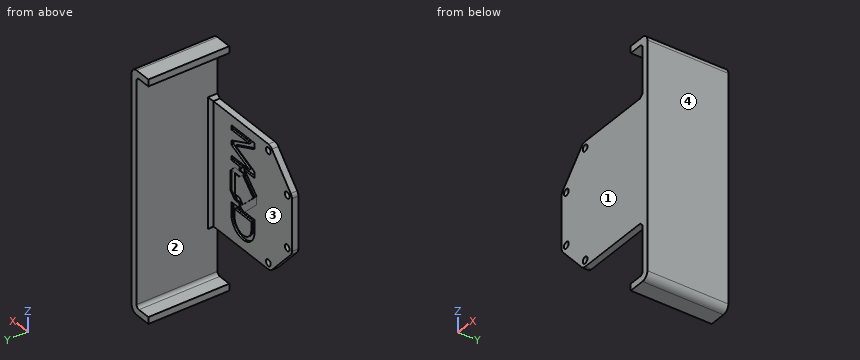
Autodesk Inventor part; units mm, degrees
ref_plane "YZ Plane" through (0, 0, 0) normal (1, 0, 0) x (0, 1, 0)
ref_plane "XZ Plane" through (0, 0, 0) normal (0, 1, 0) x (-1, 0, 0)
ref_plane "XY Plane" through (0, 0, 0) normal (0, 0, 1) x (1, 0, 0)
sketch "Sketch1" plane through (0, 0, 0) normal (0, 1, 0) x (-1, 0, 0)
  line L0 (0, 34) -> (16, 16) construction
  line L1 (18.9896, 18.6575) -> (2.9896, 36.6575)
  arc A0 (2.9896, 36.6575) -> (0, 38) centre (0, 34) ccw
  arc A1 (20, 16) -> (18.9896, 18.6575) centre (16, 16) ccw
  line L2 (16, 16) -> (16, -16) construction
  line L3 (20, -16) -> (20, 16)
  line L4 (16, -16) -> (0, -34) construction
  line L5 (2.9896, -36.6575) -> (18.9896, -18.6575)
  line L6 (0, 34) -> (-44.6053, 34) construction
  line L7 (0, 38) -> (-53, 38)
  line L8 (0, -34) -> (-49, -34) construction
  line L9 (-53, -38) -> (0, -38)
  line L10 (-49, 30.0008) -> (-49, -29.9992) construction
  line L11 (-53, 38) -> (-53, -38)
  arc A2 (18.9896, -18.6575) -> (20, -16) centre (16, -16) ccw
  arc A3 (0, -38) -> (2.9896, -36.6575) centre (0, -34) ccw
  point P0 (0, 0)
  point P1 (8, 25)
  point P2 (16, 0)
  point P3 (8, -25)
  point P4 (-24.1053, 34)
  point P5 (-24.5, -34)
  point P6 (-49, 0.0008)
  dimension "d1" = 34
  dimension "d2" = 32
  dimension "d3" = 16
  dimension "d4" = 16
  dimension "d6" = 8
  dimension "d12" = 4
  dimension "d13" = 4
  dimension "d15" = 4
  dimension "d17" = 68
  dimension "d18" = 76
  dimension "d19" = 73
  dimension "d21" = 20
  dimension "d40" = 76
  dimension "d41" = 53
extrude "Extrusion1" add sketch "Sketch1" along normal blind 4
sketch "Sketch2" plane through (0, 4, 0) normal (0, 1, 0) x (1, 0, 0)
  line L0 (-20, 16) -> (-20, -16)
  point P0 (0, 0)
  point P1 (0, -34)
  point P2 (-16, 16)
  point P3 (-16, -16)
  point P4 (0, 34)
  dimension "d31" = 34
  dimension "d33" = 20
  dimension "d34" = 16
  dimension "d35" = 4
  dimension "d36" = 16
  dimension "d37" = 4
  dimension "d38" = 20
  dimension "d39" = 34
hole "Hole1" at (0, 4, 34) at (-16, 4, -16) at (-16, 4, 16) at (0, 4, -34) direction (0, -1, 0) diameter 4 end through all
sketch "Sketch3" plane through (0, 4, 0) normal (0, 1, 0) x (1, 0, 0)
  line L0 (53, -70) -> (53, 70)
  line L1 (48.8, 70) -> (48.8, -70)
  line L2 (53, -38) -> (53, 38)
  arc A0 (53, 70) -> (48.8, 74.2) centre (48.8, 70) ccw
  arc A1 (48.8, -74.2) -> (53, -70) centre (48.8, -70) ccw
  line L3 (48.8, 74.2) -> (38.8, 74.2)
  line L4 (38.8, 74.2) -> (38.8, 70)
  line L5 (38.8, 70) -> (48.8, 70)
  line L6 (48.8, -74.2) -> (38.8, -74.2)
  line L7 (38.8, -74.2) -> (38.8, -70)
  line L8 (38.8, -70) -> (48.8, -70)
  point P0 (0, 0)
  dimension "d42" = 140
  dimension "d43" = 4.2
  dimension "d52" = 70
  dimension "d53" = 10
  dimension "d54" = 10
extrude "Extrusion2" add sketch "Sketch3" along normal blind 46 and the other way blind 4
chamfer "Chamfer1" distance 2 angle 45 3 edges at (48.8, 4, 0) (48.8, 2, 38) (48.8, 2, -38)
fillet "Fillet1" radius 2 1 edges at (48.8, 25, 70)
fillet "Fillet2" radius 2 1 edges at (48.8, 25, -70)
sketch "Sketch9" plane through (0, 4, 0) normal (0, 1, 0) x (1, 0, 0)
  line L0 (21.0218, -11.6451) -> (10.117, -0.7403)
  line L1 (10.117, -0.7403) -> (10.117, 4.4923)
  line L2 (10.117, 4.4923) -> (21.0218, 15.3971)
  line L3 (21.0218, 15.3971) -> (24.6218, 13.7645)
  line L4 (24.6218, 13.7645) -> (24.6218, 11.726)
  line L5 (24.6218, 11.726) -> (28.517, 11.726)
  line L6 (28.517, 11.726) -> (32.117, 8.126)
  line L7 (32.117, 8.126) -> (32.117, -4.374)
  line L8 (32.117, -4.374) -> (28.517, -7.974)
  line L9 (28.517, -7.974) -> (24.6218, -7.974)
  line L10 (24.6218, -7.974) -> (24.6218, -10.0125)
  line L11 (24.6218, -10.0125) -> (21.0218, -11.6451)
  line L12 (28.517, -4.374) -> (24.6218, -4.374)
  line L13 (24.6218, -4.374) -> (21.8025, -7.1932)
  line L14 (21.8025, -7.1932) -> (12.7333, 1.876)
  line L15 (12.7333, 1.876) -> (21.8025, 10.9453)
  line L16 (21.8025, 10.9453) -> (24.6218, 8.126)
  line L17 (24.6218, 8.126) -> (28.517, 8.126)
  line L18 (28.517, 8.126) -> (28.517, -4.374)
  line L19 (10.117, -0.7403) -> (24.6218, 13.7645)
  line L20 (24.6218, -10.0125) -> (10.117, 4.4923)
  line L21 (21.8025, -7.1932) -> (21.8025, 10.9453)
  line L22 (21.0218, -11.6451) -> (21.0218, 15.3971)
  line L23 (24.6218, -7.974) -> (21.0218, -7.974)
  line L24 (21.8025, -7.1932) -> (21.0218, -7.974)
  line L25 (32.117, -4.374) -> (28.517, -4.374)
  line L26 (32.117, 8.126) -> (28.517, 8.126)
  line L27 (24.6218, 11.726) -> (24.6218, 8.126)
  line L28 (28.517, 8.126) -> (28.517, 11.726)
  line L29 (21.0218, -7.974) -> (24.6218, -7.974)
  line L30 (21.8025, -7.1932) -> (21.0218, -7.974)
  line L31 (21.0218, -11.6451) -> (21.0218, -7.974)
  line L32 (12.7333, 1.876) -> (10.117, -0.7403)
  line L33 (21.8025, 10.9453) -> (24.6218, 13.7645)
  line L34 (28.517, -4.374) -> (32.117, -4.374)
  line L35 (0, -38) -> (46.8, -38)
  point P0 (-70, 0)
  point P1 (21.0218, -6.4125)
  dimension "d467" = 3.7
  dimension "d468" = 3.7
  dimension "d469" = 12.5
  dimension "d470" = 3.6
  dimension "d471" = 3.6
  dimension "d472" = 2.0385
  dimension "d473" = 3.6
  dimension "d474" = 22
  dimension "d475" = 3.6
  dimension "d523" = 30.026
extrude "Extrusion16" cut sketch "Sketch9" against normal blind 0.6 contours L22 L23 L20 L11 | L20 L23 L10 | L19 L4 L27 L16 | L25 L18 L26 L7 | L26 L28 L6
extrude "Extrusion19" cut sketch "Sketch9" against normal blind 0.3 contours L1 L20 L19 | L24 L20 L23 | L2 L22 L15 L20 | L23 L20 L13 L12 L25 L8 L9 | L3 L19 L15 L22
sketch "Sketch10" plane through (0, 4, 0) normal (0, 1, 0) x (1, 0, 0)
  line L0 (31.4873, 14.588) -> (11.8138, 14.588)
  line L1 (31.4873, 14.588) -> (31.4873, 22.6975)
  line L2 (11.8138, 22.8893) -> (11.8138, 14.588)
  line L3 (28.7873, 17.288) -> (28.7996, 22.3152)
  line L4 (28.7873, 17.288) -> (14.4873, 17.288)
  line L5 (14.4873, 17.288) -> (14.4873, 22.181)
  arc A0 (31.4873, 22.6975) -> (11.8138, 22.8893) centre (21.6443, 22.1561) ccw
  arc A1 (28.7996, 22.3152) -> (14.4873, 22.181) centre (21.6443, 22.1561) ccw
  line L6 (0, -38) -> (46.8, -38)
  line L7 (46.8, 38) -> (0, 38)
  dimension "d493" = 7.157
  dimension "d494" = 9.8579
  dimension "d495" = 2.7
  dimension "d496" = 2.6736
  dimension "d497" = 5.0272
  dimension "d498" = 19.6735
  dimension "d499" = 8.3013
  dimension "d500" = 14.3
  dimension "d520" = 19.6735
  dimension "d521" = 4.8929
  dimension "d522" = 5.986
sketch "Sketch11" plane through (0, 4, 0) normal (0, 1, 0) x (1, 0, 0)
  line L0 (16.2315, -29.314) -> (31.3715, -22.7937)
  line L1 (31.3715, -22.7937) -> (31.3715, -20.0566)
  line L2 (31.3715, -20.0566) -> (16.2315, -13.5363)
  line L3 (16.2315, -13.5363) -> (12.1356, -13.5363)
  line L4 (16.2315, -13.5363) -> (31.3715, -13.5363)
  line L5 (11.6715, -10.8363) -> (11.6715, -13.3363)
  arc A0 (12.7735, -27.8548) -> (11.6715, -29.514) centre (13.4715, -29.514) ccw
  arc A1 (11.6715, -13.3363) -> (12.773, -14.9953) centre (13.4715, -13.3363) ccw
  line L6 (12.7735, -27.8548) -> (28.0515, -21.4275)
  line L7 (12.773, -14.9953) -> (28.0515, -21.4275)
  line L8 (31.3715, -32.014) -> (11.6715, -32.014)
  line L9 (11.6715, -32.014) -> (11.6715, -29.514)
  line L10 (11.6715, -10.8363) -> (31.3715, -10.8363)
  line L11 (31.3715, -13.5363) -> (31.3715, -10.8363)
  line L12 (31.3715, -29.314) -> (16.2315, -29.314)
  line L13 (31.3715, -32.014) -> (31.3715, -29.314)
  line L14 (0, -38) -> (46.8, -38)
  line L15 (-20, 16) -> (-20, -16)
  point P0 (12.0472, -15.3794)
  dimension "d501" = 1.8
  dimension "d502" = 1.8
  dimension "d503" = 2.5
  dimension "d504" = 2.5
  dimension "d505" = 19.7
  dimension "d506" = 1.102
  dimension "d507" = 1.1016
  dimension "d509" = 15.14
  dimension "d510" = 3.32
  dimension "d511" = 2.7
  dimension "d513" = 23.3
  dimension "d514" = 23.3
  dimension "d516" = 5.986
  dimension "d517" = 19.7
  dimension "d518" = 15.14
  dimension "d519" = 31.6715
extrude "Extrusion21" cut sketch "Sketch10" against normal blind 1.2
extrude "Extrusion22" cut sketch "Sketch11" against normal blind 1.2
extrude "Extrusion23" cut sketch "Sketch9" against normal blind 0.9 contours L0 L19 L14 L22 | L27 L5 L28 L17
sketch "Sketch12" plane through (0, 2.8, 0) normal (0, 1, 0) x (1, 0, 0)
  line L0 (21.0218, -10.8363) -> (20.2129, -10.8363)
  line L1 (24.6218, -10.0125) -> (22.8052, -10.8363)
  line L2 (20.2129, -10.8363) -> (22.8052, -10.8363)
  line L3 (22.8052, -10.8363) -> (21.0218, -11.6451)
  line L4 (21.0218, -11.6451) -> (20.2129, -10.8363)
  line L5 (21.0218, -10.8363) -> (21.0218, -7.974)
  line L6 (21.0218, -10.8363) -> (21.0218, -11.6451)
  line L7 (21.0218, -6.4125) -> (21.0218, -7.974)
  line L8 (31.4873, 14.588) -> (11.8138, 14.588)
  line L9 (20.2127, 14.588) -> (22.8059, 14.588)
  line L10 (21.0218, 15.3971) -> (20.2127, 14.588)
  line L11 (22.8059, 14.588) -> (21.0218, 15.3971)
  line L12 (10.117, 4.4923) -> (20.2127, 14.588)
  line L13 (22.8059, 14.588) -> (24.6218, 13.7645)
  point P0 (0, 0)
extrude "Extrusion24" add sketch "Sketch12" along normal blind 0.9 contours L8 L10 L11
extrude "Extrusion25" add sketch "Sketch12" along normal blind 0.3 contours L6 L4 L0
extrude "Extrusion26" add sketch "Sketch12" along normal blind 0.6 contours L2 L3 L6
properties part number "pare_choc_demo_reel"
Could you check a few things on this model? Use its own coordinates, in mm. Face numbers are marked on the shaded views. A direction names the side the tool comes from. Round coordinates to 2 decimals unless told otherwise and drop trailing zeros. Loops run counter-clockwise (first coordinate to the right, second up) from the corner with the lowest first, then second, coordinate; pieces in that order, holes last. Notation, with made-up numbers: (12, 54) - (27, 54) arc R5 cw to (27, 61) - close; hole circle Ø4 at (50, 80). An arc over 180 degrees is marked (long way). Answer as CSV lines item,"result".
1. I want a section at A-A on z = 34. List the corners of the cut face in (x, y) for me.
Filled in:
outline,"(-5.35, 0) - (-2, 0) - (-2, 4) - (-5.35, 4) - close; (2, 0) - (53, 0) - (53, 50) - (48.8, 50) - (48.8, 6) - (46.8, 4) - (2, 4) - close"
2. I want a section at C-C on y = 35. List the corners of the cut face in (x, z) for me, then the cut area to 3 significant figures.
Filled in:
outline,"(38.8, -74.2) - (48.8, -74.2) arc R4.2 ccw to (53, -70) - (53, 70) arc R4.2 ccw to (48.8, 74.2) - (38.8, 74.2) - (38.8, 70) - (46.8, 70) arc R2 cw to (48.8, 68) - (48.8, -68) arc R2 cw to (46.8, -70) - (38.8, -70) - close"
area,"701 mm^2"
3. I want a section at B-B on x = -16. List the corners of the cut face in (y, z) for me.
Filled in:
outline,"(0, -22.02) - (4, -22.02) - (4, -18) - (0, -18) - close; (0, -14) - (4, -14) - (4, 14) - (0, 14) - close; (0, 18) - (4, 18) - (4, 22.02) - (0, 22.02) - close"
4. I want a section at D-D on z = -27. List the corners of the cut face in (x, y) for me, then the cut area to 3 significant figures.
Filled in:
outline,"(-11.57, 0) - (53, 0) - (53, 50) - (48.8, 50) - (48.8, 6) - (46.8, 4) - (30.23, 4) - (30.23, 2.8) - (26.91, 2.8) - (26.91, 4) - (16.38, 4) - (16.38, 2.8) - (13.06, 2.8) - (13.06, 4) - (-11.57, 4) - close"
area,"446 mm^2"
5. On a 3-axis mill with a long thin cutter (end or side, diameter ignored), from which of +Z, -Z, +X, -X, +Y, -Y can I reach the whole of each face in a straight line? I mean the marked faces 1 and 2. Say none if no direction works.
Filled in:
face 1,"+Z, -Z, +X, -X, -Y"
face 2,"-X, +Y"
6. Please list where these lines run through material, in increasing order: line 1 along Z through (x, y) = (0, 2); line 2 along X through (y, z) = (2, 16); line 3 along Z through (x, y) = (40, 19). Write a range as [from, to].
Filled in:
line 1,"z = [-38, -36], [-32, 32], [36, 38]"
line 2,"x = [-20, -18], [-14, 53]"
line 3,"z = [-74.2, -70], [70, 74.2]"
7. For pin 1 Ø1.5 at (x, z) = (35, 7) entering from +Y; pin 2 Ø1 at (x, y) = (26, 3.5) entering from -Z; pin 3 Ø1.3 at (x, y) = (26.5, 3.5) entering from +Z, each with a flat end and sliding along its axis, tell me the tip position at first contact or that it passes through.
Filled in:
pin 1,"stops at y = 4"
pin 2,"stops at z = -38"
pin 3,"stops at z = 38"
8. We'd pull the mould along Z, two halves only. Please class the marked faces 3 and 4: +Z half, -Z half, draft (parallel to the pull), parting line (faces both ways), or undercut.
Filled in:
face 3,"undercut"
face 4,"draft"
